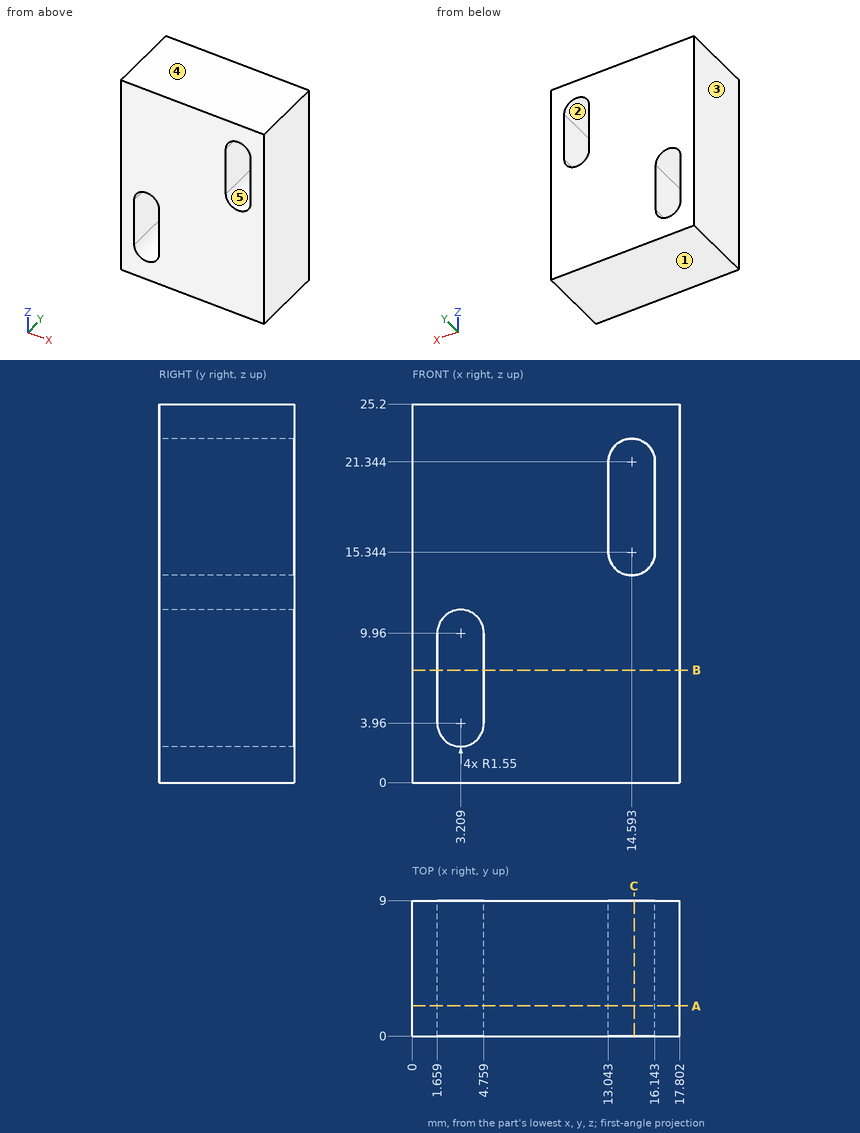
Geometry check sheet. Reference: drawing and pictorial views, mm from the part's lowest x, y, z. A direction names the side the tool comes from. Round coordinates to 2 decimals unless told otherwise and drop trailing zeros. Loops run counter-clockwise (first coordinate to the right, second up) from the corner with the lowest first, then second, coordinate; pieces in that order, holes last. Notation, with made-up numbers: M 19,-31 L 75,-31 A32 ccw 75,-4 Z; hole C -32,2.25 d10. An arc over 180 degrees is marked long. One line per item, written item: value.
(1) Sectioned sample at A-A, the plane y = 2. Record the cut outline in (x, z).
Computed values:
outline: M 0,0 L 17.8,0 L 17.8,25.2 L 0,25.2 Z; hole M 1.66,3.96 A1.55 ccw 4.76,3.96 L 4.76,9.96 A1.55 ccw 1.66,9.96 Z; hole M 13.04,15.34 A1.55 ccw 16.14,15.34 L 16.14,21.34 A1.55 ccw 13.04,21.34 Z
(2) Release check for a two-part mould opening along X. For the marked faces 3, 4 and 5 record: +X half, -X half, draft (parallel to the pull), parting line (faces both ways), or undercut.
Computed values:
face 3: -X half
face 4: draft
face 5: undercut
(3) Access from +Z, -Z, +X, -X, +Y, -Y to the whole of each face (thin tool, end or side, straight path). Record for the marked faces 1 and 2.
Computed values:
face 1: -Z, +X, -X, +Y, -Y
face 2: +Y, -Y
(4) Thickness scan on line 1 (X direction, y = 1, z = 8.75); line 2 (X direction, y = 6.25, z = 15.25) (1 decimal); line 3 (Z direction, x = 13.5, y = 5.75) (1 decimal). Record the ranges inside material, lowest first.
Computed values:
line 1: x = 0 to 1.66, 4.76 to 17.8
line 2: x = 0 to 13, 16.1 to 17.8
line 3: z = 0 to 14.2, 22.4 to 25.2
(5) Sectioned sample at B-B, the plane z = 7.5. Record the cut outline in (x, y).
Computed values:
outline: M 0,0 L 1.66,0 L 1.66,9 L 0,9 Z; M 4.76,0 L 17.8,0 L 17.8,9 L 4.76,9 Z
(6) Sectioned sample at C-C, the plane x = 14.75. Record the cut outline in (y, z).
Computed values:
outline: M 0,0 L 9,0 L 9,13.8 L 0,13.8 Z; M 0,22.89 L 9,22.89 L 9,25.2 L 0,25.2 Z
